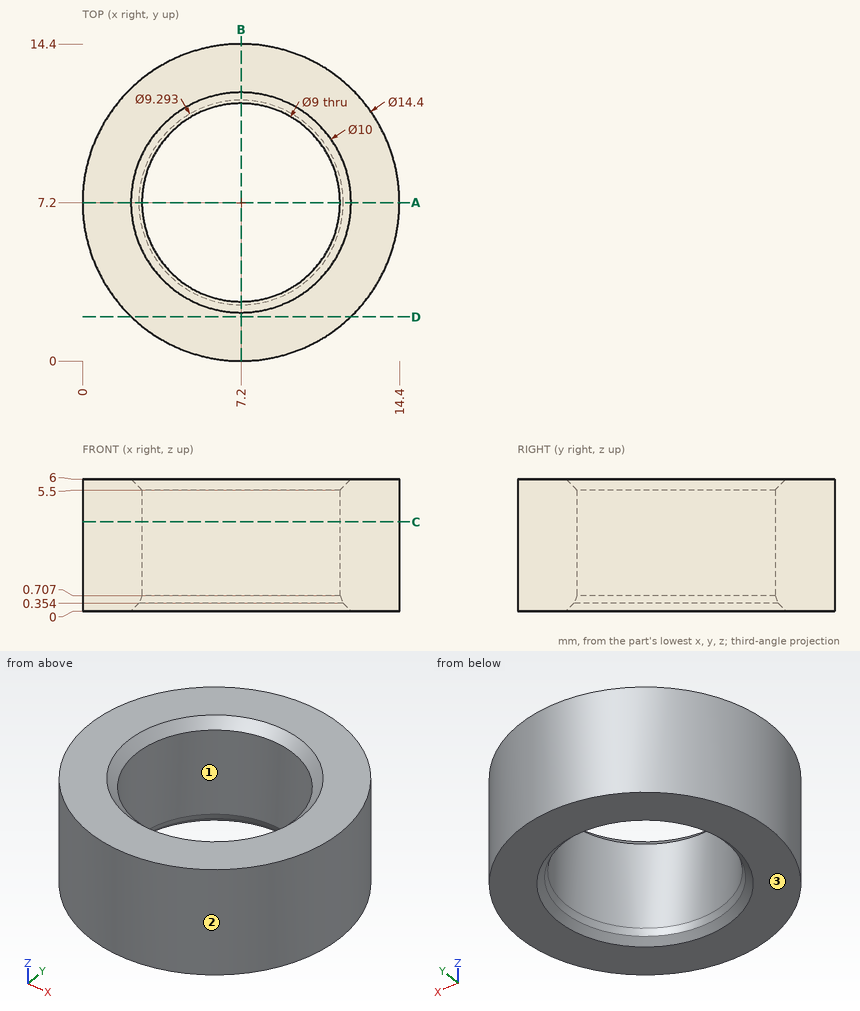
For this review, use the dimensioned drawing (mm, ordinates from the lowest corner) and the shaded views. Round coordinates to 2 decimals unless told otherwise and drop trailing zeros. Write each loop counter-clockwise with the first axis right and the second up, starting at its lowest first coordinate (ties: lowest second). Pieces come first, ordered by that corner, then holes. Notation, with made-up numbers: (-15.5, 89.5) - (39.5, 89.5) arc R24 cw to (39.5, 119.5) - close; hole circle Ø4 at (36, 10.5). An arc over 180 degrees is marked (long way). One line per item, written item: value. Start each with the question number.
1. To check wall thickness, follow L1, parallel to Y at x = 7.2, z = 4.1; L2, parallel to X at y = 9, z = 3.95 (1 decimal); L3, parallel to Y at x = 10.75, z = 2.5 (1 decimal). State the ranges of each line that lie inside material, in increasing order. Write a range as from..to.
2. Consider section D-D on y = 2. Write out the cut boundary in (x, z).
3. Consider section C-C on z = 4.05. Write out the cut boundary in (x, y).
4. Consider section A-A on y = 7.2. Write out the cut boundary in (x, z).
5. The part is to be moulded in two halves that separate along Y. For the marked faces 1, 2 and 3, say which applies: released by +Y, released by -Y, zero draft, split by the parting line, or undercut.
6. Clearance check with flat-ended pins moving along their axes: P1, Ø2, axis at x = 12.5, z = 2, coming from the +Y side (1 decimal); P2, Ø1, axis at x = 3.5, z = 2, coming from the +Y side; P3, Ø1, axis at x = 5.5, z = 3.5, coming from the +Y side; P4, Ø4, axis at x = 8, y = 5.5, coming from the +Z side. State where each tip first meets the part, or that it passes through.
Checks:
1. L1: y = 0..2.7, 11.7..14.4
1. L2: x = 0.2..3.1, 11.3..14.2
1. L3: y = 0.9..4.4, 10..13.5
2. outline: (2.22, 0) - (12.18, 0) - (12.18, 6) - (2.22, 6) - close
3. outline: circle Ø14.4 at (7.2, 7.2); hole circle Ø9 at (7.2, 7.2)
4. outline: (0, 0) - (2.2, 0) - (2.55, 0.35) - (2.7, 0.71) - (2.7, 5.5) - (2.2, 6) - (0, 6) - close; (11.7, 0.71) - (11.85, 0.35) - (12.2, 0) - (14.4, 0) - (14.4, 6) - (12.2, 6) - (11.7, 5.5) - close
5. face 1: undercut
5. face 2: split by the parting line
5. face 3: zero draft
6. P1: stops at y = 13
6. P2: stops at y = 13.65
6. P3: stops at y = 14.3
6. P4: passes through
